Check sheet for the modelled part. Datum: model origin and axes. Units: mm. Face numbers are marked on the shaded views. A direction names the side the tool comes from. Give positions to 0.01 mm unless a question says otherwise; leave off trailing zeros. Order: outer loops, then holes, each group sorted by start corner. A loop starts at its lowest first (then second) coordinate and runs counter-clockwise, first axis right, second up. Notation, with made-up numbers: M 39.25,87.25 L 77.25,87.25 A28 ccw 77.25,124.25 Z; hole C 35.5,70.25 d6. An arc over 180 degrees is marked long. Answer in a Markdown table with one row per item. Add a question column.
from build123d import *

# Parameters (mm, degrees)
BOSS_EXTRUDE1_DEPTH = 4.5
CUT_EXTRUDE1_DEPTH  = 2.5
CUT_EXTRUDE2_DEPTH  = 0.414110472
CUT_EXTRUDE3_DEPTH  = 0.414110472
CUT_EXTRUDE4_DEPTH  = 0.385889528
CUT_EXTRUDE5_DEPTH  = 0.385889528
CUT_EXTRUDE6_DEPTH  = 0.33137085
CUT_EXTRUDE7_DEPTH  = 0.33137085
CUT_EXTRUDE8_DEPTH  = 0.254269796
SKETCH10_W          = 5
SKETCH10_H          = 2
CUT_EXTRUDE9_DEPTH  = 0.214359354
CUT_EXTRUDE10_DEPTH = 0.254269796
SKETCH12_W          = 5
SKETCH12_H          = 2
CUT_EXTRUDE11_DEPTH = 0.214359354
SKETCH13_W          = 4.5
SKETCH13_H          = 3.2
CUT_EXTRUDE12_DEPTH = 25
BOSS_EXTRUDE2_DEPTH = 2
CUT_EXTRUDE13_DEPTH = 39.14773912
DRAFT1_START        = -2
DRAFT1_DEPTH        = 4.5
DRAFT1_2_DEPTH      = 2.5
DRAFT1_3_DEPTH      = 2


# Read off the part's stored shape, not the designer's step: Draft1
with BuildPart() as part:
    # Sketch1 → Boss-Extrude1 (new body)
    with BuildSketch(Plane(origin=(0, 0, -2), x_dir=(-1, 0, 0), z_dir=(0, 0, -1))):
        Polygon((-33, 12.160106278), (-33, 7.839893722), (-32.781925288, 6.743558111), (-32.512829008, 5.950826033), (-32.142562584, 5.2), (-31.677461378, 4.503926854), (-31.1254834, 3.8745166), (-30.496073146, 3.322538622), (-29.8, 2.857437416), (-29.049173967, 2.487170992), (-28.256441889, 2.218074712), (-27.43536763, 2.054752887), (-26.6, 2), (-1.4, 2), (-0.56463237, 2.054752887), (0.256441889, 2.218074712), (1.049173967, 2.487170992), (1.8, 2.857437416), (2.496073146, 3.322538622), (3.1254834, 3.8745166), (3.677461378, 4.503926854), (4.142562584, 5.2), (4.512829008, 5.950826033), (4.781925288, 6.743558111), (4.945247113, 7.56463237), (5, 8.4), (5, 11.6), (4.945247113, 12.43536763), (4.781925288, 13.256441889), (4.512829008, 14.049173967), (4.142562584, 14.8), (3.677461378, 15.496073146), (3.1254834, 16.1254834), (2.496073146, 16.677461378), (1.8, 17.142562584), (1.049173967, 17.512829008), (0.256441889, 17.781925288), (-0.56463237, 17.945247113), (-1.4, 18), (-26.6, 18), (-27.43536763, 17.945247113), (-28.256441889, 17.781925288), (-29.049173967, 17.512829008), (-29.8, 17.142562584), (-30.496073146, 16.677461378), (-31.1254834, 16.1254834), (-31.677461378, 15.496073146), (-32.142562584, 14.8), (-32.512829008, 14.049173967), (-32.781925288, 13.256441889), align=None)
    extrude(amount=-BOSS_EXTRUDE1_DEPTH)

    # Sketch2 → Cut-Extrude1 (cut)
    with BuildSketch(Plane.XY.offset(2.5)):
        Polygon((29.6, 10), (29.545481322, 10.414110472), (29.385640646, 10.8), (29.13137085, 11.13137085), (28.8, 11.385640646), (28.414110472, 11.545481322), (28, 11.6), (28, 8.4), (28.414110472, 8.454518678), (28.8, 8.614359354), (29.13137085, 8.86862915), (29.385640646, 9.2), (29.545481322, 9.585889528), align=None)
    extrude(amount=-CUT_EXTRUDE1_DEPTH, mode=Mode.SUBTRACT)

    # Sketch3 → Cut-Extrude2 (cut)
    with BuildSketch(Plane.XZ.offset(-10)):
        Polygon((28, 0), (28, -2), (33, -2), (33, 0), (29.545481322, 0), align=None)
    extrude(amount=-CUT_EXTRUDE2_DEPTH, mode=Mode.SUBTRACT)

    # Sketch4 → Cut-Extrude3 (cut)
    with BuildSketch(Plane(origin=(0, 10, 0), x_dir=(-1, 0, 0), z_dir=(0, 1, 0))):
        Polygon((-28, -2), (-28, 0), (-29.545481322, 0), (-33, 0), (-33, -2), align=None)
    extrude(amount=-CUT_EXTRUDE3_DEPTH, mode=Mode.SUBTRACT)

    # Sketch5 → Cut-Extrude4 (cut)
    with BuildSketch(Plane.XZ.offset(-10.414110472)):
        Polygon((28, 0), (28, -2), (33, -2), (33, 0), (29.385640646, 0), align=None)
    extrude(amount=-CUT_EXTRUDE4_DEPTH, mode=Mode.SUBTRACT)

    # Sketch6 → Cut-Extrude5 (cut)
    with BuildSketch(Plane(origin=(0, 9.585889528, 0), x_dir=(-1, 0, 0), z_dir=(0, 1, 0))):
        Polygon((-28, -2), (-28, 0), (-29.385640646, 0), (-33, 0), (-33, -2), align=None)
    extrude(amount=-CUT_EXTRUDE5_DEPTH, mode=Mode.SUBTRACT)

    # Sketch7 → Cut-Extrude6 (cut)
    with BuildSketch(Plane.XZ.offset(-10.8)):
        Polygon((28, 0), (28, -2), (33, -2), (33, 0), (29.13137085, 0), align=None)
    extrude(amount=-CUT_EXTRUDE6_DEPTH, mode=Mode.SUBTRACT)

    # Sketch8 → Cut-Extrude7 (cut)
    with BuildSketch(Plane(origin=(0, 9.2, 0), x_dir=(-1, 0, 0), z_dir=(0, 1, 0))):
        Polygon((-28, -2), (-28, 0), (-29.13137085, 0), (-33, 0), (-33, -2), align=None)
    extrude(amount=-CUT_EXTRUDE7_DEPTH, mode=Mode.SUBTRACT)

    # Sketch9 → Cut-Extrude8 (cut)
    with BuildSketch(Plane.XZ.offset(-11.13137085)):
        Polygon((28, 0), (28, -2), (33, -2), (33, 0), (28.8, 0), align=None)
    extrude(amount=-CUT_EXTRUDE8_DEPTH, mode=Mode.SUBTRACT)

    # Sketch10 → Cut-Extrude9 (cut)
    with BuildSketch(Plane.XZ.offset(-11.385640646)):
        with Locations((30.5, -1)):
            Rectangle(SKETCH10_W, SKETCH10_H)
    extrude(amount=-CUT_EXTRUDE9_DEPTH, mode=Mode.SUBTRACT)

    # Sketch11 → Cut-Extrude10 (cut)
    with BuildSketch(Plane(origin=(0, 8.86862915, 0), x_dir=(-1, 0, 0), z_dir=(0, 1, 0))):
        Polygon((-28, -2), (-28, 0), (-28.8, 0), (-33, 0), (-33, -2), align=None)
    extrude(amount=-CUT_EXTRUDE10_DEPTH, mode=Mode.SUBTRACT)

    # Sketch12 → Cut-Extrude11 (cut)
    with BuildSketch(Plane(origin=(0, 8.614359354, 0), x_dir=(-1, 0, 0), z_dir=(0, 1, 0))):
        with Locations((-30.5, -1)):
            Rectangle(SKETCH12_W, SKETCH12_H)
    extrude(amount=-CUT_EXTRUDE11_DEPTH, mode=Mode.SUBTRACT)

    # Sketch13 → Cut-Extrude12 (cut)
    with BuildSketch(Plane(origin=(28, 0, 0), x_dir=(0, 0, -1), z_dir=(1, 0, 0))):
        with Locations((-0.25, 10)):
            Rectangle(SKETCH13_W, SKETCH13_H)
    extrude(amount=-CUT_EXTRUDE12_DEPTH, mode=Mode.SUBTRACT)

    # Sketch14 → Boss-Extrude2 (add)
    with BuildSketch(Plane.XY.offset(2.5)):
        Polygon((1.674873734, 12.474873734), (2.231088913, 11.75), (2.580740392, 10.905866658), (2.7, 10), (2.580740392, 9.094133342), (2.231088913, 8.25), (1.674873734, 7.525126266), (0.95, 6.968911087), (0.105866658, 6.619259608), (-0.8, 6.5), (-1.705866658, 6.619259608), (-2.55, 6.968911087), (-3.274873734, 7.525126266), (-3.831088913, 8.25), (-4.180740392, 9.094133342), (-4.3, 10), (-4.180740392, 10.905866658), (-3.831088913, 11.75), (-3.274873734, 12.474873734), (-2.55, 13.031088913), (-1.705866658, 13.380740392), (-0.8, 13.5), (0.105866658, 13.380740392), (0.95, 13.031088913), align=None)
    extrude(amount=BOSS_EXTRUDE2_DEPTH)

    # Sketch15 → Cut-Extrude13 (cut, through all)
    with BuildSketch(Plane(origin=(0, 0, -2), x_dir=(-1, 0, 0), z_dir=(0, 0, -1))):
        Polygon((-0.938666487, 9.534125719), (-0.758845727, 9.1), (-0.472792206, 8.727207794), (-0.1, 8.441154273), (0.334125719, 8.261333513), (0.8, 8.2), (1.265874281, 8.261333513), (1.7, 8.441154273), (2.072792206, 8.727207794), (2.358845727, 9.1), (2.538666487, 9.534125719), (2.6, 10), (2.538666487, 10.465874281), (2.358845727, 10.9), (2.072792206, 11.272792206), (1.7, 11.558845727), (1.265874281, 11.738666487), (0.8, 11.8), (0.334125719, 11.738666487), (-0.1, 11.558845727), (-0.472792206, 11.272792206), (-0.758845727, 10.9), (-0.938666487, 10.465874281), (-1, 10), align=None)
    extrude(amount=-CUT_EXTRUDE13_DEPTH, mode=Mode.SUBTRACT)

    # Draft1 outline → Draft1 (cut)
    with BuildSketch(Plane.XY.offset(DRAFT1_START)):
        Polygon((33, 8.399999998), (32.945247113, 7.56463237), (33, 7.839893722), align=None)
    extrude(amount=DRAFT1_DEPTH, mode=Mode.SUBTRACT)

    # Draft1 2 outline → Draft1 2 (add)
    with BuildSketch(Plane.XY):
        Polygon((33, 8.399999998), (33.185369442, 11.228191161), (33, 12.160106278), align=None)
    extrude(amount=DRAFT1_2_DEPTH)

    # Draft1 3 outline → Draft1 3 (add)
    with BuildSketch(Plane.XY.offset(DRAFT1_START)):
        Polygon((33, 12.160106278), (33, 11.6), (33.111412066, 11.6), align=None)
    extrude(amount=DRAFT1_3_DEPTH)


solid = part.part
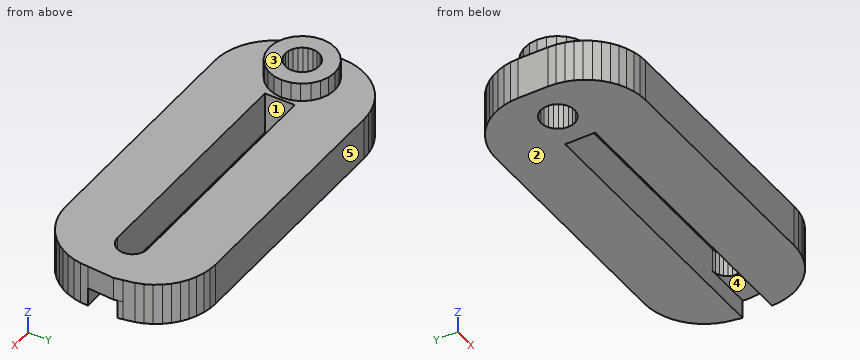
Q1. Draft check along Y on the marked faces 3, 4 and 5. Enter one of: pulls with the +Y half, pulls with the -Y half, needs draft (parallel to the pull), parting line crosses it, or undercut.
Q2. Go/stop test with flat-tipped pins: pin 1 (1.5 mm diameter, centred on y = 11.5, z = 3.5, fed in from -X); pin 2 (1 mm diameter, centred on x = 30, y = 10, fed in from -Z). Record where each tip stops, or that it passes through.
Q3. Cross-section at C-C (x = 27). Record the boundary of the cut face in (y, z).
Q4. Cross-section at A-A (x = 17). Record the boundary of the cut face in (y, z).
Q5. Thickness scan on probe 1 along Y at (x, z) = (5.5, 0.5); probe 2 along Y at (x, z) = (-2, 1); probe 3 along Z at (x, y) = (-2, 14.5). Record the ranges inside material, lowest first.
Q6. Cross-section at B-B (z = 0.75). State how many separate pieces and enclosed holes the cut face has, and give its area (3 significant figures).
Q7. Tool access check on the marked faces 1 and 2. Record the directions out of +Z, -Z, +X, -X, +Y, -Y that give a thin tool (end or side, any length) a straight path to the whole face; none if there is none.
Values follow:
| question | item | result |
|---|---|---|
| 1 | face 3 | needs draft |
| 1 | face 4 | undercut |
| 1 | face 5 | pulls with the +Y half |
| 2 | pin 1 | x = -4.2 |
| 2 | pin 2 | z = 0 |
| 3 | outline | M 2.03,-2 L 8.4,-2 L 8.4,2.5 L 2.03,2.5 Z; M 11.6,-2 L 17.97,-2 L 17.97,2.5 L 11.6,2.5 Z |
| 4 | outline | M 2,-2 L 8.4,-2 L 8.4,2.5 L 2,2.5 Z; M 11.6,-2 L 18,-2 L 18,2.5 L 11.6,2.5 Z |
| 5 | probe 1 | 2 to 8.4, 11.6 to 18 |
| 5 | probe 2 | 2.99 to 8.67, 11.33 to 17.01 |
| 5 | probe 3 | -2 to 2.5 |
| 6 | separate pieces | 1 |
| 6 | enclosed holes | 2 |
| 6 | area | 479 mm² |
| 7 | face 1 | +Z, -Z |
| 7 | face 2 | -Z, +X, -X, +Y, -Y |
